Build history of the part. All positions in model axes, mm. Face numbers are marked on the shaded views. A direction names the side the tool comes from. Round coordinates to 2 decimals unless told otherwise and drop trailing zeros. Write each loop counter-clockwise with the first axis right and the second up, starting at its lowest first coordinate (ties: lowest second). Pieces come first, ordered by that corner, then holes. Notation, with made-up numbers: M 62,18 L 94,18 A7 ccw 94,26 Z; hole C -1,13 d6. An arc over 180 degrees is marked long. Write item = value, one per line.
from build123d import *

# Parameters (mm, degrees)
CROQUIS1_R              = 3.5
SALIENTE_EXTRUIR1_DEPTH = 11
CORTAR_EXTRUIR1_DEPTH   = 7
CROQUIS4_R              = 1.15
CORTAR_EXTRUIR2_DEPTH   = 2.3


with BuildPart() as part:
    # Croquis1 → Saliente-Extruir1 (new body)
    with BuildSketch(Plane.XY):
        Circle(CROQUIS1_R)
    extrude(amount=SALIENTE_EXTRUIR1_DEPTH)

    # Croquis3 → Cortar-Extruir1 (cut)
    with BuildSketch(Plane(origin=(0, 0, 0), x_dir=(-1, 0, 0), z_dir=(0, 0, -1))):
        Polygon((1.549659556, 2.684875278), (-1.550340419, 2.684482182), (-3.099999975, -0.000393096), (-1.549659556, -2.684875278), (1.550340419, -2.684482182), (3.099999975, 0.000393096), align=None)
    extrude(amount=-CORTAR_EXTRUIR1_DEPTH, mode=Mode.SUBTRACT)

    # Croquis4 → Cortar-Extruir2 (cut)
    with BuildSketch(Plane.XY.offset(11)):
        Circle(CROQUIS4_R)
    extrude(amount=-CORTAR_EXTRUIR2_DEPTH, mode=Mode.SUBTRACT)


solid = part.part
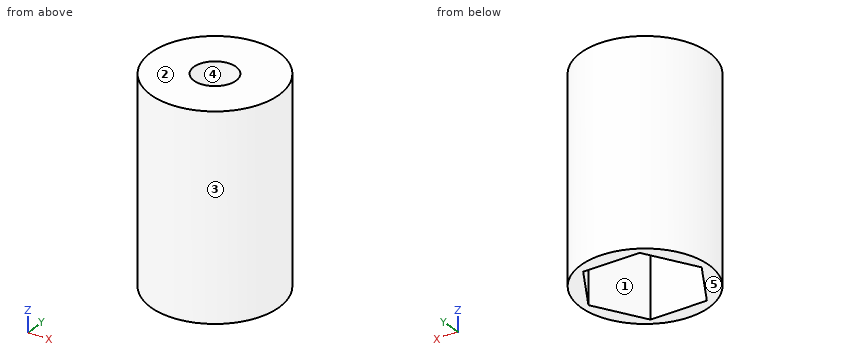
1. Flat gauge pins, fed straight in: pin 1 (1 mm diameter, centred on x = -2.5, z = 1.5, fed in from +Y); pin 2 (2 mm diameter, centred on y = -2.5, z = 3.5, fed in from +X); pin 3 (3 mm diameter, centred on x = 0, y = -1, fed in from -Z). Where does each tip first touch, or does it go through?
Responses:
pin_1 = 2.87
pin_2 = 3.16
pin_3 = 7
2. Mould opens along X. For the marked faces 3, 4 and 5 say: pulls with the +X half, pulls with the -X half, needs draft (parallel to the pull), parting line crosses it, or undercut.
Responses:
face_3 = parting line crosses it
face_4 = undercut
face_5 = needs draft
3. Band-saw the part on C-C (y = -0.25). List the corners of the cut face in (x, z), plus the area to 3 significant figures.
Responses:
outline = M -3.49,0 L -2.96,0 L -2.96,7 L 2.96,7 L 2.96,0 L 3.49,0 L 3.49,11 L 1.12,11 L 1.12,8.7 L -1.12,8.7 L -1.12,11 L -3.49,11 Z
area = 30.3 mm²
4. Probe probe 1 along Y at (x, z) = (0, 9.75); probe 2 along X at (y, z) = (-0.75, 4.25); probe 3 along Y at (x, z) = (-0.75, 9.5). List the from-to ranges inside material, lowest first.
Responses:
probe_1 = -3.5 to -1.15, 1.15 to 3.5
probe_2 = -3.42 to -2.67, 2.67 to 3.42
probe_3 = -3.42 to -0.87, 0.87 to 3.42
5. Tool access for the marked faces 1 and 2: list every direction of +Z, -Z, +X, -X, +Y, -Y with a clear straight run to the whole face (end or side of a thin tool).
Responses:
face_1 = -Z
face_2 = +Z, +X, -X, +Y, -Y
6. Band-saw the part on D-D (z = 7.75). List the corners of the cut face in (x, y).
Responses:
outline = C 0,0 d7
7. Band-saw the part on B-B (x = -2). List the corners of the cut face in (y, z), plus the area to 3 significant figures.
Responses:
outline = M -2.87,0 L -1.91,0 L -1.91,7 L 1.91,7 L 1.91,0 L 2.87,0 L 2.87,11 L -2.87,11 Z
area = 36.5 mm²
8. Band-saw the part on A-A (z = 6.5). List the corners of the cut face in (x, y).
Responses:
outline = C 0,0 d7; hole M -3.1,0 L -1.55,-2.68 L 1.55,-2.68 L 3.1,0 L 1.55,2.68 L -1.55,2.68 Z
